```python
from build123d import *

# Parameters (mm, degrees)
ESBO_O1_R                  = 5
ESBO_O1_R_2                = 4
RESSALTO_EXTRUS_O1_DEPTH   = 400
CORTE_EXTRUS_O1_DEPTH      = 401.062495118
CORTE_EXTRUS_O1_DEPTH_BACK = 401.062495118
ESBO_O2_R                  = 1.6


with BuildPart() as part:
    # Esboço1 → Ressalto-extrusão1 (new body)
    with BuildSketch(Plane(origin=(0, 0, 0), x_dir=(1, 0, 0), z_dir=(0, 1, 0))):
        with Locations(Location((0, 0, 0), (0, 0, 270))):
            Circle(ESBO_O1_R)
        with Locations(Location((0, 0, 0), (0, 0, 270))):
            Circle(ESBO_O1_R_2, mode=Mode.SUBTRACT)
    extrude(amount=RESSALTO_EXTRUS_O1_DEPTH)

    # Esboço2 → Corte-extrusão1 (cut, two sides: drawn at the far end of the back side and taken through both)
    with BuildSketch(Plane.XY.offset(-CORTE_EXTRUS_O1_DEPTH_BACK)):
        with Locations((0, 236.5)):
            Circle(ESBO_O2_R)
        with Locations((0, 163.5)):
            Circle(ESBO_O2_R)
    extrude(amount=CORTE_EXTRUS_O1_DEPTH + CORTE_EXTRUS_O1_DEPTH_BACK, mode=Mode.SUBTRACT)


solid = part.part
```
Verification items for the finished model (mm, model axes). Coordinates: 2 decimals unless noted, no trailing zeros. Loops run counter-clockwise (first coordinate to the right, second up) from the corner with the lowest first, then second, coordinate; pieces in that order, holes last. Notation, with made-up numbers: (47.5, 30) -> (51.5, 30) arc R25 cw to (51.5, 58) -> close; hole circle Ø4 at (81, 64.5). An arc over 180 degrees is marked (long way). Answer in a Markdown table with one row per item. Add a question column.
1. Draft check along Z on faces 1 (the face through (-4.88, 197.2, -1.08)), 2 (the face through (-3.905, 197.2, -0.867)). Enter one of: +Z half, -Z half, draft (parallel to the pull), parting line (faces both ways), or undercut.
2. Depth check by flat-ended pin: P1, Ø1, axis at x = -3.5, y = 354.5, coming from the +Z side; P2, Ø2, axis at x = 3, y = 345, coming from the -Z side; P3, Ø5, axis at x = 3.5, y = 81, coming from the +Z side. Enter the tip coordinate at first touch or a pass-through.
3. Section check A-A, the plane z = 0. Enter the section's corners in (x, y).
4. Material ranges on probe 1 along Y at (x, z) = (0, 4.7); probe 2 along X at (y, z) = (38, 0), recorded low to high. Write a range as [from, to].
5. Section check B-B, the plane x = 0. Enter the section's corners in (y, z), then the cut area to 3 significant figures.
6. Section check C-C, the plane y = 306. Enter the section's corners in (x, z), then the cut area to 3 significant figures.
Derived:
| question | item | result |
|---|---|---|
| 1 | face 1 | parting line |
| 1 | face 2 | undercut |
| 2 | P1 | stops at z = 4 |
| 2 | P2 | stops at z = -4.58 |
| 2 | P3 | stops at z = 4.9 |
| 3 | outline | (-5, 0) -> (-4, 0) -> (-4, 400) -> (-5, 400) -> close; (4, 0) -> (5, 0) -> (5, 400) -> (4, 400) -> close |
| 4 | probe 1 | y = [0, 161.9], [165.1, 234.9], [238.1, 400] |
| 4 | probe 2 | x = [-5, -4], [4, 5] |
| 5 | outline | (0, -5) -> (161.9, -5) -> (161.9, -4) -> (0, -4) -> close; (0, 4) -> (161.9, 4) -> (161.9, 5) -> (0, 5) -> close; (165.1, -5) -> (234.9, -5) -> (234.9, -4) -> (165.1, -4) -> close; (165.1, 4) -> (234.9, 4) -> (234.9, 5) -> (165.1, 5) -> close; (238.1, -5) -> (400, -5) -> (400, -4) -> (238.1, -4) -> close; (238.1, 4) -> (400, 4) -> (400, 5) -> (238.1, 5) -> close |
| 5 | area | 787 mm² |
| 6 | outline | circle Ø10 at (0, 0); hole circle Ø8 at (0, 0) |
| 6 | area | 28.3 mm² |
